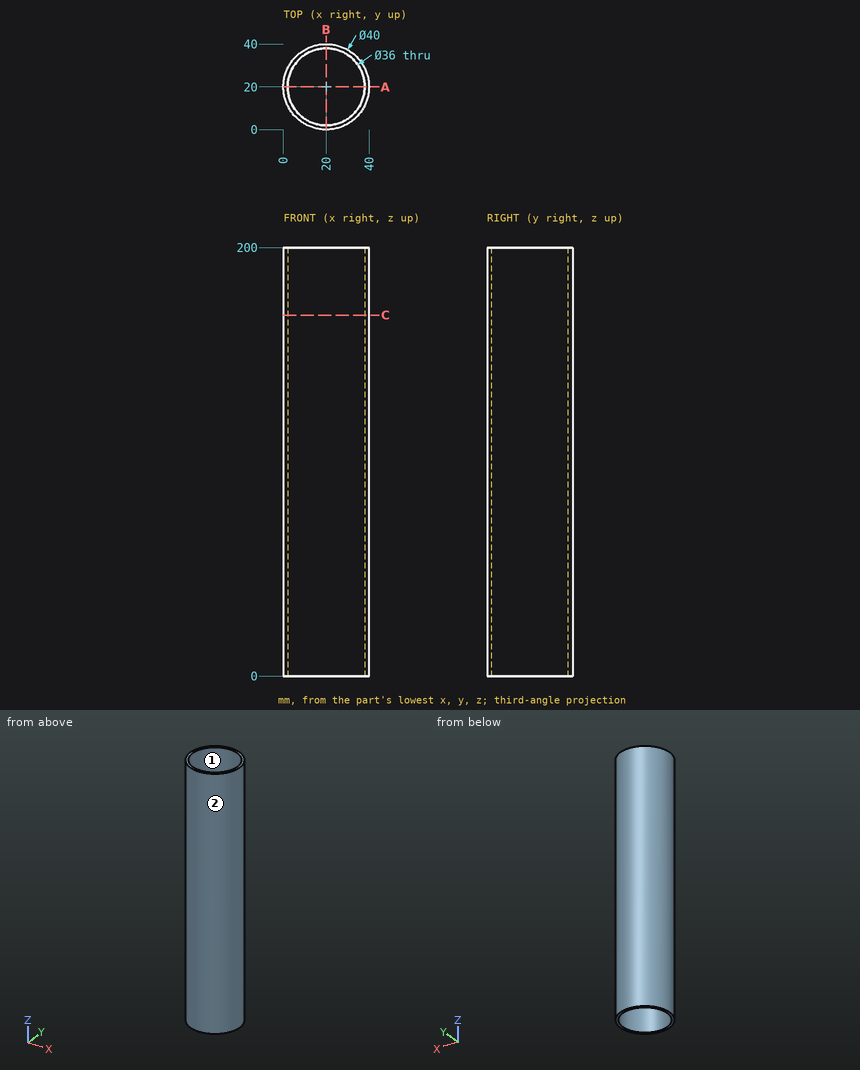
Verification items for this drawing (mm, ordinates from the low corner). Coordinates: 2 decimals unless noted, no trailing zeros. Write each loop counter-clockwise with the first axis right and the second up, starting at its lowest first coordinate (ties: lowest second). Pieces come first, ordered by that corner, then holes. Notation, with made-up numbers: M 78.5,-0.75 L 113.5,-0.75 A22 cw 113.5,26.25 Z; hole C 68.5,-10 d9. An arc over 180 degrees is marked long. Use CSV: the item, a comma, the result in double quotes.
Q1. Section check C-C, the plane z = 168.5. Enter the section's corners in (x, y).
Computed values:
outline,"C 20,20 d40; hole C 20,20 d36"
Q2. Mould release check, pull along Y, two halves, no side actions. Record for the marked faces 1 and 2: pulls with the +Y half, pulls with the -Y half, needs draft (parallel to the pull), parting line crosses it, or undercut.
Computed values:
face 1,"undercut"
face 2,"parting line crosses it"
Q3. Section check A-A, the plane y = 20. Enter the section's corners in (x, z).
Computed values:
outline,"M 0,0 L 2,0 L 2,200 L 0,200 Z; M 38,0 L 40,0 L 40,200 L 38,200 Z"
Q4. Thickness scan on line 1 along X through (y, z) = (20, 64.5); line 2 along Y through (x, z) = (31, 46); line 3 along Y through (x, z) = (32.5, 137). Record the ranges inside material, lowest first. Write a range as [from, to].
Computed values:
line 1,"[0, 2], [38, 40]"
line 2,"[3.3, 5.75], [34.25, 36.7]"
line 3,"[4.39, 7.05], [32.95, 35.61]"
Q5. Go/stop test with flat-tipped pins: P1, Ø3, axis at x = 32.5, z = 147, coming from the -Y side; P2, Ø6, axis at x = 34.5, z = 110.5, coming from the +Y side; P3, Ø2, axis at x = 22.5, z = 104, coming from the +Y side. Record where each tip stops, or that it passes through.
Computed values:
P1,"y = 3.3"
P2,"y = 36.36"
P3,"y = 39.94"
